from build123d import *

# Parameters (mm, degrees)
F0_R         = 11
F0_R_2       = 9
F0_R_3       = 3.25
F1_DEPTH     = 12
F2_R         = 8.5
F2_R_2       = 3.25
F3_DEPTH     = 10
F0_R_4       = 13
F1_FACE1_R   = 11
F1_FACE1_R_2 = 3.25
F4_DEPTH     = 2


with BuildPart() as f1:
    # F0 (on Right) → F1 (new body)
    with BuildSketch(Plane.YZ):
        Circle(F0_R)
        Circle(F0_R_2, mode=Mode.SUBTRACT)
        Circle(F0_R_2)
        Circle(F0_R_3, mode=Mode.SUBTRACT)
    extrude(amount=F1_DEPTH)

    # F2 (on face) → F3 (cut)
    with BuildSketch(Plane.YZ.offset(12)):
        Circle(F2_R)
        Circle(F2_R_2, mode=Mode.SUBTRACT)
    extrude(amount=-F3_DEPTH, mode=Mode.SUBTRACT)

    # F0 (on Right) + F1_face1 (on face) → F4 (join)
    with BuildSketch(Plane.YZ):
        Circle(F0_R_4)
        Circle(F0_R, mode=Mode.SUBTRACT)
        Circle(F0_R)
        Circle(F0_R_2, mode=Mode.SUBTRACT)
        Circle(F0_R_2)
        Circle(F0_R_3, mode=Mode.SUBTRACT)
    with BuildSketch(Plane(origin=(0, 0, 0), x_dir=(0, 1, 0), z_dir=(-1, 0, 0))):
        Circle(F1_FACE1_R)
        Circle(F1_FACE1_R_2, mode=Mode.SUBTRACT)
    extrude(amount=F4_DEPTH, dir=(1, 0, 0))


solid = f1.part
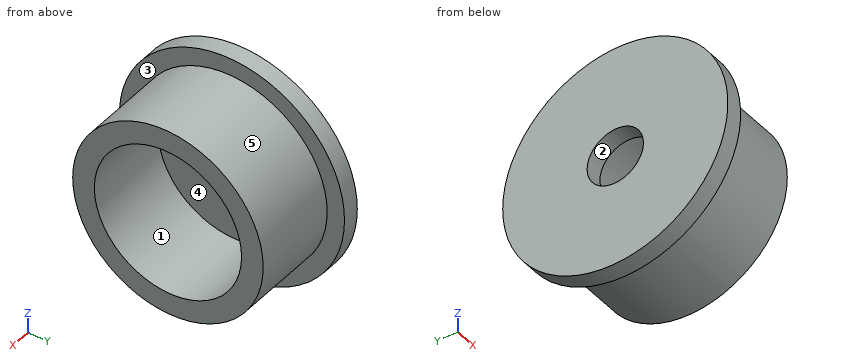
Can you work these out from the model? Positions are in its coordinate system, mm. Face numbers are marked on the shaded views. A direction names the side the tool comes from. Give positions to 0.01 mm unless a question says otherwise; leave off trailing zeros. Write each loop counter-clockwise with the first axis right and the second up, starting at its lowest first coordinate (ties: lowest second). Pieces come first, ordered by that corner, then holes. Notation, with made-up numbers: M 34,-12.5 L 39,-12.5 A7 ccw 39,-0.5 Z; hole C 69,31 d10. An arc over 180 degrees is marked long. Answer in a Markdown table with one row per item. Add a question column.
Item 1: Imagine slicing it at D-D, the plane x = 3.75. Write out the boundary of the cut face in (y, z).
Item 2: On a 3-axis mill with a long thin cutter (end or side, diameter ignored), from which of +Z, -Z, +X, -X, +Y, -Y can I reach the whole of each face in a straight line? I mean the marked faces 1 and 2. Say none if no direction works.
Item 3: Please list where these lines run through material, in increasing order: L1, parallel to Z at x = 1.65, y = 0; L2, parallel to Z at x = 5, y = 0; L3, parallel to X at y = 4.25, z = -1.25.
Item 4: For pin 1 Ø1.5 at (x, y) = (3, -3) entering from +Z; pin 2 Ø2 at (y, z) = (9, 3.5) entering from -X; pin 3 Ø6 at (x, y) = (8.5, 7) entering from +Z; pin 4 Ø5 at (y, z) = (1.5, 3.5) entering from +X, each with a flat end and sliding along its axis, tell me the tip position at first contact or that it passes through.
Item 5: Imagine slicing it at A-A, the plane y = 0. Write out the boundary of the cut face in (x, z).
Item 6: Imagine slicing it at C-C, the plane z = -9. Write out the boundary of the cut face in (x, y).
Item 7: We'd pull the mould along Y, two halves only. Please class the marked faces 3, 4 and 5: released by +Y, released by -Y, zero draft, split by the parting line, or undercut.
Evaluation:
| question | item | result |
|---|---|---|
| 1 | outline | C 0,0 d22; hole C 0,0 d17 |
| 2 | face 1 | +X |
| 2 | face 2 | +X, -X |
| 3 | L1 | z = -13 to -3.25, 3.25 to 13 |
| 3 | L2 | z = -11 to -8.5, 8.5 to 11 |
| 3 | L3 | x = 0 to 2 |
| 4 | pin 1 | stops at z = 10.77 |
| 4 | pin 2 | stops at x = 0 |
| 4 | pin 3 | stops at z = 10.25 |
| 4 | pin 4 | stops at x = 2 |
| 5 | outline | M 0,-13 L 2,-13 L 2,-11 L 12,-11 L 12,-8.5 L 2,-8.5 L 2,-3.25 L 0,-3.25 Z; M 0,3.25 L 2,3.25 L 2,8.5 L 12,8.5 L 12,11 L 2,11 L 2,13 L 0,13 Z |
| 6 | outline | M 0,-9.38 L 2,-9.38 L 2,-6.32 L 12,-6.32 L 12,6.32 L 2,6.32 L 2,9.38 L 0,9.38 Z |
| 7 | face 3 | zero draft |
| 7 | face 4 | undercut |
| 7 | face 5 | split by the parting line |
